Read the model definition and answer for the solid it produces. Units are mm, in the model's axes. A direction names the side the tool comes from. Coordinates: 2 decimals unless noted, no trailing zeros. Loops run counter-clockwise (first coordinate to the right, second up) from the corner with the lowest first, then second, coordinate; pieces in that order, holes last. Notation, with made-up numbers: M 54,73.5 L 97,73.5 A28 cw 97,109.5 Z; hole C 16,1 d6. An arc over 180 degrees is marked long. One line per item, written item: value. Start each with the question number.
```python
from build123d import *

# Parameters (mm, degrees)
CUT_EXTRUDE1_DEPTH = 1


with BuildPart() as part:
    # Sketch1 → Revolve1 (revolve)
    with BuildSketch(Plane(origin=(0, 0, 0), x_dir=(0, 0, -1), z_dir=(1, 0, 0)), mode=Mode.PRIVATE) as revolve1_sk:
        with BuildLine():
            Line((0, 0), (0, 1.7))
            Line((0, 1.7), (0.2, 1.9))
            Line((0.2, 1.9), (1.84, 1.9))
            Line((1.84, 1.9), (2, 1.74))
            Line((2, 1.74), (2, 1.3))
            ThreePointArc((2, 1.3), (2.015193643, 1.24701055), (2.056157637, 1.210123155))
            Line((2.056157637, 1.210123155), (2.466157637, 1.010123155))
            ThreePointArc((2.466157637, 1.010123155), (2.48750205, 1.00256365), (2.51, 1))
            Line((2.51, 1), (7.8, 1))
            Line((7.8, 1), (8, 0.8))
            Line((8, 0.8), (8, 0))
            Line((8, 0), (0, 0))
        make_face()
    revolve(revolve1_sk.sketch.rotate(Axis((0, 0, 0), (0, 0, -1)), 90), axis=Axis((0, 0, 0), (0, 0, -1)))

    # Sketch2 → Cut-Extrude1 (cut)
    with BuildSketch(Plane.XY):
        Polygon((0, 0.866025404), (-0.75, 0.433012702), (-0.75, -0.433012702), (0, -0.866025404), (0.75, -0.433012702), (0.75, 0.433012702), align=None)
    extrude(amount=-CUT_EXTRUDE1_DEPTH, mode=Mode.SUBTRACT)

    # Sketch3 → Cut-Revolve2 (revolve, cut)
    with BuildSketch(Plane(origin=(0, 0, 0), x_dir=(0, 0, -1), z_dir=(1, 0, 0)), mode=Mode.PRIVATE) as cut_revolve2_sk:
        Polygon((1, 0), (1, 0.75), (1.433012702, 0), align=None)
    revolve(cut_revolve2_sk.sketch.rotate(Axis((0, 0, -1), (0, 0, -1)), 90), axis=Axis((0, 0, -1), (0, 0, -1)), mode=Mode.SUBTRACT)

    # Sketch4 → Cut-Revolve3 (revolve, cut)
    with BuildSketch(Plane(origin=(0, 0, 0), x_dir=(0, 0, -1), z_dir=(1, 0, 0))):
        Polygon((0, 0.866025404), (0, 0.75), (0.031088913, 0.75), align=None)
    revolve(axis=Axis((0, 0, 0), (0, 0, -1)), mode=Mode.SUBTRACT)


solid = part.part
```
1) A tool of negligible diameter and unlimited length cuts with its end or side. For faces 4 (the face through (0.75, 0, -0.5)), 5 (the face through (0, 1, -5)), 6 (the face through (0, 0, -8)), from which of +Z, -Z, +X, -X, +Y, -Y can it reach the whole face along a straight path? Write none if from no direction.
2) Flat-ended cylindrical pins translate along their axes: pin 1 (1 mm diameter, centred on x = -0.5, y = 1, fed in from -Z); pin 2 (1.5 mm diameter, centred on x = 1, y = -1.5, fed in from -Z); pin 3 (2 mm diameter, centred on y = 0.5, z = -5.5, fed in from +X). Find the tip coordinate at first contact, or state that the pin passes through.
3) Section A-A (z = -5.75) is taken. Determine the outline of the cut face in (x, y).
4) For a pull along Y with two mould halves and no side action, classify faces 1 (the face through (-1, 1, 0)), 2 (the face through (-0.75, 0, -0.5)), 3 (the face through (1.812, -0.571, -1.031)) as released by +Y, released by -Y, zero draft, split by the parting line, or undercut.
5) Consider line 1 along Y through (x, z) = (-0.05, -7.25); line 2 along X through (y, z) = (0.75, -0.75); line 3 along Z through (x, y) = (-0.25, 1.45). Determine where each line is inside the solid, lowest interval first.
6) Section B-B (z = -1.25) is taken. Determine the outline of the cut face in (x, y).
Results found:
1. face 4: +Z
1. face 5: -Z
1. face 6: -Z, +X, -X, +Y, -Y
2. pin 1: stops at z = -8
2. pin 2: stops at z = -2.38
2. pin 3: stops at x = 1
3. outline: C 0,0 d2
4. face 1: zero draft
4. face 2: undercut
4. face 3: split by the parting line
5. line 1: y = -1 to 1
5. line 2: x = -1.75 to -0.2, 0.2 to 1.75
5. line 3: z = -2 to 0
6. outline: C 0,0 d3.8; hole C 0,0 d0.63
